Autodesk Inventor part; units mm, degrees
ref_plane "YZ Plane" through (0, 0, 0) normal (1, 0, 0) x (0, 1, 0)
ref_plane "XZ Plane" through (0, 0, 0) normal (0, 1, 0) x (-1, 0, 0)
ref_plane "XY Plane" through (0, 0, 0) normal (0, 0, 1) x (1, 0, 0)
sketch "Эскиз1" plane through (0, 0, 0) normal (0, 0, 1) x (1, 0, 0)
  line L0 (2.3094, 4) -> (4.6188, 0)
  line L1 (4.6188, 0) -> (2.3094, -4)
  line L2 (2.3094, -4) -> (-2.3094, -4)
  line L3 (-2.3094, -4) -> (-4.6188, 0)
  line L4 (-4.6188, 0) -> (-2.3094, 4)
  line L5 (-2.3094, 4) -> (2.3094, 4)
  circle A0 centre (0, 0) radius 2.5
  dimension "d0" = 8
  dimension "d3" = 5
extrude "Выдавливание1" add sketch "Эскиз1" along normal blind 3 contours L0 L1 L2 L3 L4 L5 | A0
extrude "Выдавливание2" add sketch "Эскиз1" against normal blind 15 contours A0
thread "Резьба1"
properties part number "Болт"
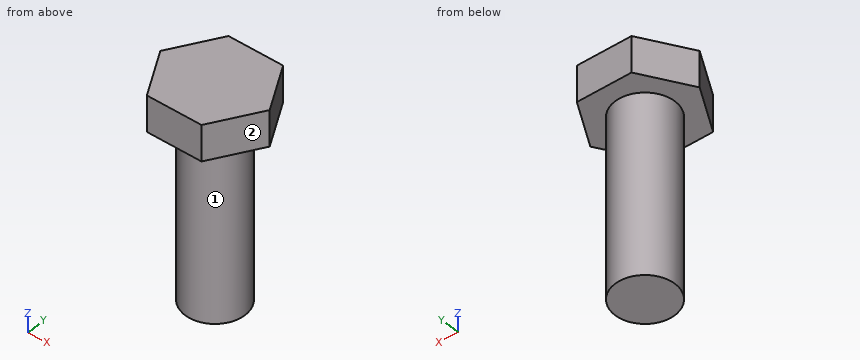
For this review, take the finished solid that the model builds, in its own axes (mm). Face numbers are marked on the shaded views. A direction names the side the tool comes from. Round coordinates to 2 decimals unless told otherwise and drop trailing zeros. Write each loop counter-clockwise with the first axis right and the second up, starting at its lowest first coordinate (ties: lowest second). Pieces come first, ordered by that corner, then holes. Notation, with made-up numbers: M 88.25,-23.75 L 95.25,-23.75 A16 cw 95.25,3.25 Z; hole C -32,80 d6. An arc over 180 degrees is marked long. One line per item, written item: value. Start each with the question number.
(1) Insertion check: pin 1 (2 mm diameter, centred on y = -2.5, z = -13, fed in from +X); pin 2 (1 mm diameter, centred on x = -0.5, z = -1.5, fed in from +Y); pin 3 (5 mm diameter, centred on x = -1, z = -5.5, fed in from -Y). Each pin has a flat end and moves straight along its axis. Give the tip position at first contact, or say it passes through.
(2) Wall thickness on line 1 (Z direction, x = -0.25, y = 3); line 2 (X direction, y = 0.5, z = 0.25); line 3 (X direction, y = 1.75, z = -2.5): over which ranges is each line inside the solid? List them lowest first.
(3) We need section B-B (y = -2.25). Give the boundary of the cut face in (x, z).
(4) We need section C-C (y = 3.75). Give the boundary of the cut face in (x, z).
(5) Machinability: for the marked faces 1 and 2, which of the approach directions +Z, -Z, +X, -X, +Y, -Y give a long, thin tool a straight path to every point of the face, cutting with its end or side? Answer none if there is none.
(6) We need section A-A (x = 0). Give the boundary of the cut face in (y, z), and give its area (3 significant figures).
(7) We need section D-D (x = -4). Give the boundary of the cut face in (y, z).
Result:
1. pin 1: x = 2
1. pin 2: y = 2.5
1. pin 3: y = -2.5
2. line 1: 0 to 3
2. line 2: -4.33 to 4.33
2. line 3: -1.79 to 1.79
3. outline: M -3.32,0 L -1.09,0 L -1.09,-15 L 1.09,-15 L 1.09,0 L 3.32,0 L 3.32,3 L -3.32,3 Z
4. outline: M -2.45,0 L 2.45,0 L 2.45,3 L -2.45,3 Z
5. face 1: -Z
5. face 2: +Z, -Z, +X, -Y
6. outline: M -4,0 L -2.5,0 L -2.5,-15 L 2.5,-15 L 2.5,0 L 4,0 L 4,3 L -4,3 Z
6. area: 99.0 mm²
7. outline: M -1.07,0 L 1.07,0 L 1.07,3 L -1.07,3 Z
